Model file for the job. Use its own axes, mm. Face numbers are marked on the shaded views. A direction names the side the tool comes from. Give positions to 0.01 mm unless a question says otherwise; leave off trailing zeros. Write each loop counter-clockwise with the first axis right and the second up, starting at its lowest first coordinate (ties: lowest second). Pieces come first, ordered by that corner, then holes. Notation, with made-up numbers: (84.5, 81.5) - (118.5, 81.5) arc R19 ccw to (118.5, 106.5) - close; hole circle Ø5 at (36, -28). An arc over 180 degrees is marked (long way). Use a Markdown table: item, result. Add a question column.
```python
from build123d import *

# Parameters (mm, degrees)
PAD_DEPTH    = 0.4
SKETCH001_R  = 2.25
PAD001_DEPTH = 3.5
FILLET_R     = 1


with BuildPart() as part:
    # Sketch → Pad (new body)
    with BuildSketch(Plane.XY):
        with BuildLine():
            ThreePointArc((-2.745826, 0.625), (-8.68, 0), (-2.745826, -0.625))
            Line((-2.745826, -0.625), (2.745826, -0.625))
            ThreePointArc((2.745826, -0.625), (5.68, -3), (8.614174, -0.625))
            Line((8.614174, -0.625), (14.105826, -0.625))
            ThreePointArc((14.105826, -0.625), (20.04, 0), (14.105826, 0.625))
            Line((8.614174, 0.625), (14.105826, 0.625))
            ThreePointArc((8.614174, 0.625), (5.68, 3), (2.745826, 0.625))
            Line((-2.745826, 0.625), (2.745826, 0.625))
        make_face()
    extrude(amount=PAD_DEPTH)

    # Sketch001 → Pad001 (join)
    with BuildSketch(Plane.XY):
        with Locations((-5.68, 0)):
            Circle(SKETCH001_R)
        with Locations((5.68, 0)):
            Circle(SKETCH001_R)
        with Locations((17.04, 0)):
            Circle(SKETCH001_R)
    extrude(amount=PAD001_DEPTH)

    # Fillet
    fillet_edges = [part.edges().sort_by_distance(p)[0] for p in [
        (-7.93, 0, 3.5),
        (3.43, 0, 3.5),
        (14.79, 0, 3.5),
    ]]
    fillet(fillet_edges, radius=FILLET_R)


solid = part.part
```
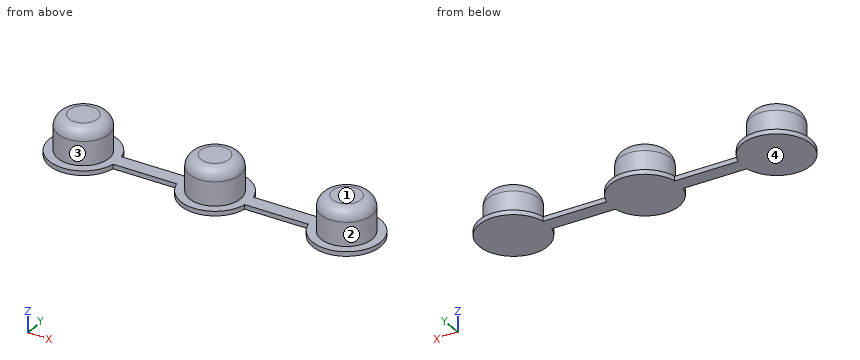
(1) Band-saw the part on D-D (x = -1). Write the cut outline in (y, z) (3 decimals).
(2) Which spindle directions (+Z, -Z, +X, -X, +Y, -Y) get a long thin tool onto all of the face, cutting with end or side? Do the marked faces 1 and 2. Say none if no direction does.
(3) Two-plate mould, pull along X, no slides. Class the marked faces 3 and 4: +X half, -X half, draft (parallel to the pull), parting line (faces both ways), or undercut.
(4) Flat gauge pins, fed straight in: pin 1 (2 mm diameter, centred on y = 1, z = 3, fed in from +X); pin 2 (1.5 mm diameter, centred on x = 16.5, z = 3, fed in from -Y). Where does each tip first touch, or does it go through?
(5) Band-saw the part on B-B (z = 1.05). Write the cut outline in (x, y).
(6) Band-saw the part on C-C (y = 0). Write the cut outline in (x, z), then the cut area to 3 significant figures.
(7) Probe probe 1 along X at (y, z) = (-1.5, 2.7); probe 2 along X at (y, z) = (1.5, 1.6); probe 3 along Z at (x, y) = (-4, 2). List the from-to ranges inside material, lowest first. Write a range as [from, to].
(8) Band-saw the part on A-A (x = -5.68). Write the cut outline in (y, z).
Model answer:
| question | item | result |
|---|---|---|
| 1 | outline | (-0.625, 0) - (0.625, 0) - (0.625, 0.4) - (-0.625, 0.4) - close |
| 2 | face 1 | +Z, +X, -X, +Y, -Y |
| 2 | face 2 | +Z |
| 3 | face 3 | undercut |
| 3 | face 4 | draft |
| 4 | pin 1 | stops at x = 19.29 |
| 4 | pin 2 | stops at y = -2.25 |
| 5 | outline | circle Ø4.5 at (-5.68, 0); circle Ø4.5 at (5.68, 0); circle Ø4.5 at (17.04, 0) |
| 6 | outline | (-8.68, 0) - (20.04, 0) - (20.04, 0.4) - (19.29, 0.4) - (19.29, 2.5) arc R1 ccw to (18.29, 3.5) - (15.79, 3.5) arc R1 ccw to (14.79, 2.5) - (14.79, 0.4) - (7.93, 0.4) - (7.93, 2.5) arc R1 ccw to (6.93, 3.5) - (4.43, 3.5) arc R1 ccw to (3.43, 2.5) - (3.43, 0.4) - (-3.43, 0.4) - (-3.43, 2.5) arc R1 ccw to (-4.43, 3.5) - (-6.93, 3.5) arc R1 ccw to (-7.93, 2.5) - (-7.93, 0.4) - (-8.68, 0.4) - close |
| 6 | area | 52.1 mm^2 |
| 7 | probe 1 | x = [-7.33, -4.03], [4.03, 7.33], [15.39, 18.69] |
| 7 | probe 2 | x = [-7.36, -4], [4, 7.36], [15.36, 18.72] |
| 7 | probe 3 | z = [0, 0.4] |
| 8 | outline | (-3, 0) - (3, 0) - (3, 0.4) - (2.25, 0.4) - (2.25, 2.5) arc R1 ccw to (1.25, 3.5) - (-1.25, 3.5) arc R1 ccw to (-2.25, 2.5) - (-2.25, 0.4) - (-3, 0.4) - close |
